from build123d import *

# Parameters (mm, degrees)
SKETCH001_R       = 1.58
POCKET_DEPTH      = 0.001
POCKET_DEPTH_BACK = -12.001


with BuildPart() as part:
    # Sketch → Revolution (revolve)
    with BuildSketch(Plane.XZ):
        Polygon((-16, 7), (-12, 10), (-12, 12), (-18, 12), (-18, 3), (-26.05, 3), (-26.05, 0), (-16, 0), align=None)
    revolve(axis=Axis((0, 0, 0), (0, 0, 1)))

    # Sketch001 → Pocket (cut, two sides)
    with BuildSketch(Plane.XY) as pocket_sk:
        with Locations((22.47, 0)):
            Circle(SKETCH001_R)
        with Locations((0, -22.47)):
            Circle(SKETCH001_R)
        with Locations((-15.888689, -15.888689)):
            Circle(SKETCH001_R)
        with Locations((15.888689, 15.888689)):
            Circle(SKETCH001_R)
    extrude(amount=-POCKET_DEPTH, mode=Mode.SUBTRACT)
    extrude(pocket_sk.sketch, amount=-POCKET_DEPTH_BACK, mode=Mode.SUBTRACT)


solid = part.part
Work out the finished part from the listing and answer in its coordinate system (mm). A direction names the side the tool comes from. Give positions to 0.01 mm unless a question says otherwise; leave off trailing zeros. Write each loop counter-clockwise with the first axis right and the second up, starting at its lowest first coordinate (ties: lowest second). Pieces come first, ordered by that corner, then holes. Notation, with made-up numbers: M 69,82 L 116,82 A17 cw 116,98 Z; hole C 8,68.25 d6. An arc over 180 degrees is marked long. Answer as CSV lines item,"result".
Q1. A cutting plane is placed at B-B on y = 0. Write down the section's boundary in (x, z).
A:
outline,"M -26.05,0 L -16,0 L -16,7 L -12,10 L -12,12 L -18,12 L -18,3 L -26.05,3 Z; M 12,10 L 16,7 L 16,0 L 20.89,0 L 20.89,3 L 18,3 L 18,12 L 12,12 Z; M 24.05,0 L 26.05,0 L 26.05,3 L 24.05,3 Z"
Q2. Find the intervals of material crossed by probe 1 along X at (y, z) = (0, 2); probe 2 along Y at (x, z) = (0, 3.5); probe 3 along Y at (x, z) = (0, 11.45), in increasing order. Write a range as [from, to].
A:
probe 1,"x = [-26.05, -16], [16, 20.89], [24.05, 26.05]"
probe 2,"y = [-18, -16], [16, 18]"
probe 3,"y = [-18, -12], [12, 18]"
Q3. A cutting plane is placed at D-D on x = 22.47. Write down the section's boundary in (y, z), plus the area to 3 significant figures.
A:
outline,"M -13.18,0 L -1.58,0 L -1.58,3 L -13.18,3 Z; M 1.58,0 L 13.18,0 L 13.18,3 L 1.58,3 Z"
area,"69.6 mm²"
Q4. A cutting plane is placed at A-A on x = 0. Write down the section's boundary in (y, z).
A:
outline,"M -26.05,0 L -24.05,0 L -24.05,3 L -26.05,3 Z; M -20.89,0 L -16,0 L -16,7 L -12,10 L -12,12 L -18,12 L -18,3 L -20.89,3 Z; M 12,10 L 16,7 L 16,0 L 26.05,0 L 26.05,3 L 18,3 L 18,12 L 12,12 Z"
Q5. A cutting plane is placed at C-C on z = 6. Write down the section's boundary in (x, y).
A:
outline,"C 0,0 d36; hole C 0,0 d32"
Q6. Given P1, Ø1.5, axis at x = 11.5, z = 5, coming from the +Y side; P2, Ø6, axis at y = 11, z = 6.5, coming from the +X side; P3, Ø10, axis at x = 6.5, y = -7.5, coming from the +Z side; P4, Ø1.5, axis at y = 16.5, z = 4.5, coming from the -X side, each flat-ended and moving along its own axis, determine where each tip first touches the part or whether it passes through.
A:
P1,"stops at y = 14.44"
P2,"stops at x = 16.12"
P3,"stops at z = 12"
P4,"stops at x = -8.71"
Q7. The mould has two halves that part along X. Classify faces 4 (the flat face through (4, 12, 12)), 5 (the cylindrical face through (20.672, 15.851, 1.479)), 6 (the cylindrical face through (14.31, 15.96, 1.48)): +X half, -X half, draft (parallel to the pull), parting line (faces both ways), or undercut.
A:
face 4,"draft"
face 5,"parting line"
face 6,"undercut"
Q8. A tool of negligible diameter and unlimited length cuts with its end or side. For faces 1 (the cylindrical face through (3.47, 15.62, 3.55)), 2 (the cylindrical face through (11.99, -0.53, 11.01)), 3 (the flat face through (-18, 5, 3)), from which of +Z, -Z, +X, -X, +Y, -Y can it reach the whole face along a straight path? Write none if from no direction.
A:
face 1,"-Z"
face 2,"+Z, -Z"
face 3,"+Z"
